Could you check a few things on this model? Use its own coordinates, in mm. A direction names the side the tool comes from. Give positions to 0.01 mm unless a question says otherwise; leave off trailing zeros. Loops run counter-clockwise (first coordinate to the right, second up) from the corner with the lowest first, then second, coordinate; pieces in that order, holes last. Notation, with made-up numbers: M 71.25,74 L 78.25,74 A9 ccw 78.25,89 Z; hole C -30.75,-30.75 d1. An arc over 180 degrees is marked long. Return JSON: item names as keys, results as strings. Group by question number.
1. For pin 1 (19 mm diameter, centred on x = 0, y = 7, fed in from -Z), with a flat end and sliding along its axis, tell me the tip position at first contact or that it passes through.
2. If we section it at A-A (z = 10.5): Write out the boundary of the cut face in (x, y) (1 decimal), plus the area to 3 significant figures.
3. For faces 1 (the flat face through (-1, -26.988, -4)), 2 (the flat face through (-1, -20.638, -4)), which set-ups out of +Z, -Z, +X, -X, +Y, -Y let a thin tool reach every point of the face, with its end or its side?
4. Please list where these lines run through material, in increasing order: line 1 (Y direction, x = 49.5, z = 3); line 2 (Z direction, x = -6.5, y = -16.5); line 3 (Z direction, x = -1, y = -23).
5. If we section it at C-C (y = 5): Write out the boundary of the cut face in (x, z) (1 decimal).
```python
from build123d import *

# Parameters (mm, degrees)
SKETCH1_W           = 184.15
SKETCH1_H           = 53.975
BOSS_EXTRUDE1_DEPTH = 23.8125
FILLET1_R           = 7.9375
SHELL1_T            = -6.35


with BuildPart() as part:
    # Sketch1 → Boss-Extrude1 (new, symmetric)
    with BuildSketch(Plane.XY):
        Rectangle(SKETCH1_W, SKETCH1_H)
    extrude(amount=BOSS_EXTRUDE1_DEPTH, both=True)

    # Fillet1
    fillet1_edges = [part.edges().sort_by_distance(p)[0] for p in [
        (0, 26.9875, 23.8125),
        (0, -26.9875, 23.8125),
    ]]
    fillet(fillet1_edges, radius=FILLET1_R)

    # Shell1
    shell1_openings = [part.faces().sort_by_distance(p)[0] for p in [
        (0, 0, -23.8125),
        (92.075, 0, -0.234313972),
        (-92.075, 0, -0.234313972),
    ]]
    offset(amount=SHELL1_T, openings=shell1_openings, kind=Kind.INTERSECTION)


solid = part.part
```
Answer:
{
 "1": {"pin 1": "stops at z = 17.46"},
 "2": {"outline": "M -92.1,-27 L 92.1,-27 L 92.1,-20.6 L -92.1,-20.6 Z; M -92.1,20.6 L 92.1,20.6 L 92.1,27 L -92.1,27 Z", "area": "2,340 mm²"},
 "3": {"face 1": "+Z, -Z, +X, -X, -Y", "face 2": "-Z, +X, -X"},
 "4": {"line 1": "y = -26.99 to -20.64, 20.64 to 26.99", "line 2": "z = 17.46 to 23.81", "line 3": "z = -23.81 to 22.76"},
 "5": {"outline": "M -92.1,17.5 L 92.1,17.5 L 92.1,23.8 L -92.1,23.8 Z"}
}
